from build123d import *

# Parameters (mm, degrees)
IZIM1_W                       = 15
IZIM1_H                       = 15
Y_KSEKLIK_EKSTR_ZYON1_DEPTH   = 125
Y_KSEKLIK_EKSTR_ZYON1_2_DEPTH = 125
Y_KSEKLIK_EKSTR_ZYON4_DEPTH   = 5
Y_KSEKLIK_EKSTR_ZYON5_REACH   = 179.359
IZIM6_W                       = 15
IZIM6_H                       = 15
IZIM7_R                       = 11
KES_EKSTR_ZYON2_DEPTH         = 53


with BuildPart() as part:
    # izim1 → Y_kseklik-Ekstr_zyon1 (new body)
    with BuildSketch(Plane.XY):
        with Locations((7.5, 7.5)):
            Rectangle(IZIM1_W, IZIM1_H)
    extrude(amount=Y_KSEKLIK_EKSTR_ZYON1_DEPTH)



with BuildPart() as body_2:
    # izim1 → Y_kseklik-Ekstr_zyon1 2 (new body)
    with BuildSketch(Plane.XY):
        with Locations((87.5, 7.5)):
            Rectangle(IZIM1_W, IZIM1_H)
    extrude(amount=Y_KSEKLIK_EKSTR_ZYON1_2_DEPTH)


with BuildPart() as part_1:
    add(part.part)

    add(body_2.part)  # Y_kseklik-Ekstr_zyon4 merges body 2
    # izim3 → Y_kseklik-Ekstr_zyon4 (add, symmetric)
    with BuildSketch(Plane(origin=(0, 0, 0), x_dir=(-1, 0, 0), z_dir=(0, 0, -1))):
        Polygon((-95, 67.5), (-100, 67.5), (-100, 42.5), (-95, 42.5), (-95, 15), (-80, 15), (-80, 42.5), (-15, 42.5), (-15, 0), (0, 0), (0, 42.5), (5, 42.5), (5, 67.5), (0, 67.5), (-15, 67.5), (-80, 67.5), align=None)
    extrude(amount=Y_KSEKLIK_EKSTR_ZYON4_DEPTH, both=True)

    # izim6 → Y_kseklik-Ekstr_zyon5 (add, up to next)
    with BuildSketch(Plane(origin=(0, 0, -5), x_dir=(-1, 0, 0), z_dir=(0, 0, -1)), mode=Mode.PRIVATE) as y_kseklik_ekstr_zyon5_sk1:
        with Locations((-87.5, 7.5)):
            Rectangle(IZIM6_W, IZIM6_H)
    y_kseklik_ekstr_zyon5_tool1 = extrude(y_kseklik_ekstr_zyon5_sk1.sketch, amount=-Y_KSEKLIK_EKSTR_ZYON5_REACH, mode=Mode.PRIVATE) - part_1.part
    add(y_kseklik_ekstr_zyon5_tool1.solids().sort_by_distance((87.5, 7.5, -5))[0])

    # izim7 → Kes-Ekstr_zyon2 (cut)
    with BuildSketch(Plane(origin=(0, 0, -5), x_dir=(-1, 0, 0), z_dir=(0, 0, -1))):
        with Locations((-47.5, 55)):
            Circle(IZIM7_R)
    extrude(amount=-KES_EKSTR_ZYON2_DEPTH, mode=Mode.SUBTRACT)


solid = part_1.part
Part model, mm, in its own coordinate system. A direction names the side the tool comes from. Coordinates: 2 decimals unless noted, no trailing zeros. Order: outer loops, then holes, each group sorted by start corner. A loop starts at its lowest first (then second) coordinate and runs counter-clockwise, first axis right, second up.
(1) Slice it at A-A, the plane y = 19.5. Write the cut outline in (x, z).
Check sheet entries:
outline: (0, -5) - (15, -5) - (15, 5) - (0, 5) - close; (80, -5) - (95, -5) - (95, 5) - (80, 5) - close
(2) Probe L1, parallel to X at y = 8.5, z = 109; L2, parallel to Y at x = 47, z = 0; L3, parallel to Z at x = 20, y = 63.5. List the from-to ranges inside material, lowest first.
Check sheet entries:
L1: x = 0 to 15, 80 to 95
L2: y = 42.5 to 44.01, 65.99 to 67.5
L3: z = -5 to 5
(3) Pull direction X, two halves, no side cores. Call faces 1 (the face through (15, 12, 45)), 2 (the face through (37, 47, 5)), 3 (the face through (0, 12, 45)): pulls with the +X half, pulls with the -X half, needs draft (parallel to the pull), parting line crosses it, or undercut.
Check sheet entries:
face 1: undercut
face 2: needs draft
face 3: pulls with the -X half
(4) Slice it at D-D, the plane x = 28. Write the cut outline in (y, z).
Check sheet entries:
outline: (42.5, -5) - (67.5, -5) - (67.5, 5) - (42.5, 5) - close
(5) Tool access for faces 4 (the face through (7, 15, 64)), 5 (the face through (95, 12, 45)), 6 (the face through (80, 12, 45)), 7 (the face through (8, 0, 59)), 8 (the face through (-2, 42.5, 0)): list every direction of +Z, -Z, +X, -X, +Y, -Y with a clear straight run to the whole face (end or side of a thin tool).
Check sheet entries:
face 4: +Z, +X, -X, +Y
face 5: +Z, -Z, +X, -Y
face 6: +Z, -Z, -Y
face 7: +Z, -Z, +X, -X, -Y
face 8: +Z, -Z, -X, -Y
(6) Pin check, flat tips, straight feed: pin 1 Ø4 at (x, z) = (97.5, -2) entering from -Y; pin 2 Ø4.5 at (x, z) = (84.5, 49) entering from +Y; pin 3 Ø2 at (y, z) = (11, 65.5) entering from +X. Stop position of each tip, or through.
Check sheet entries:
pin 1: stops at y = 42.5
pin 2: stops at y = 15
pin 3: stops at x = 95
(7) Slice it at C-C, the plane x = 12.5. Write the cut outline in (y, z).
Check sheet entries:
outline: (0, -5) - (67.5, -5) - (67.5, 5) - (15, 5) - (15, 125) - (0, 125) - close
(8) Slice it at B-B, the plane x = 47.5. Write the cut outline in (y, z), and give its area (3 significant figures).
Check sheet entries:
outline: (42.5, -5) - (44, -5) - (44, 5) - (42.5, 5) - close; (66, -5) - (67.5, -5) - (67.5, 5) - (66, 5) - close
area: 30.0 mm2
